```python
from build123d import *

# Parameters (mm, degrees)
SKETCH1_R                = 0.406598389
SKETCH1_R_2              = 1.143
BASE_EXTRUDE_DEPTH       = 6.35
SKETCH2_W                = 2.8702
SKETCH2_H                = 3.81
CUT_EXTRUDE1_DEPTH       = 33.262756347
SKETCH3_W                = 3.302
SKETCH3_H                = 0.508
BOSS_EXTRUDE1_DEPTH      = 3.81
BOSS_EXTRUDE2_DEPTH      = 3.81
SKETCH5_W                = 6.170551723
SKETCH5_H                = 2.54
CUT_EXTRUDE2_DEPTH       = 6.096
SKETCH6_R                = 2.3114
BOSS_EXTRUDE3_DEPTH      = 2.54
BOSS_EXTRUDE4_DEPTH      = 0.254
BOSS_EXTRUDE4_DEPTH_BACK = 4.064
SKETCH7_R                = 0.752584906


with BuildPart() as part:
    # Sketch1 → Base-Extrude (new body)
    with BuildSketch(Plane.XY):
        with BuildLine():
            Line((15.748192067, 1.405399301), (15.748192067, 10.955799301))
            Line((15.748192067, 10.955799301), (15.240192067, 11.463799301))
            Line((15.240192067, 11.463799301), (15.240192067, 14.079999301))
            Line((15.240192067, 14.079999301), (13.131992067, 14.079999301))
            ThreePointArc((13.131992067, 14.079999301), (12.5931767, 14.303183934), (12.369992067, 14.841999301))
            Line((12.369992067, 14.841999301), (12.369992067, 19.718799301))
            ThreePointArc((12.369992067, 19.718799301), (12.5931767, 20.257614668), (13.131992067, 20.480799301))
            Line((13.131992067, 20.480799301), (23.876192067, 20.480799301))
            ThreePointArc((23.876192067, 20.480799301), (24.415007435, 20.257614668), (24.638192067, 19.718799301))
            Line((24.638192067, 19.718799301), (24.638192067, 1.405399301))
            ThreePointArc((24.638192067, 1.405399301), (24.415007435, 0.866583934), (23.876192067, 0.643399301))
            Line((23.876192067, 0.643399301), (16.510192067, 0.643399301))
            ThreePointArc((16.510192067, 0.643399301), (15.9713767, 0.866583934), (15.748192067, 1.405399301))
        make_face()
        with Locations((13.639992067, 18.270999301)):
            Circle(SKETCH1_R, mode=Mode.SUBTRACT)
        with Locations((13.639992067, 15.095999301)):
            Circle(SKETCH1_R, mode=Mode.SUBTRACT)
        with Locations((22.275992067, 5.799599301)):
            Circle(SKETCH1_R_2, mode=Mode.SUBTRACT)
        with BuildLine():
            Line((23.418992067, 15.197599301), (23.418992067, 15.451599301))
            ThreePointArc((23.418992067, 15.451599301), (22.275992067, 16.594599301), (21.132992067, 15.451599301))
            Line((21.132992067, 15.451599301), (21.132992067, 15.197599301))
            ThreePointArc((21.132992067, 15.197599301), (22.275992067, 14.054599301), (23.418992067, 15.197599301))
        make_face(mode=Mode.SUBTRACT)
    extrude(amount=-BASE_EXTRUDE_DEPTH)

    # Sketch2 → Cut-Extrude1 (cut, through all)
    with BuildSketch(Plane(origin=(0, 20.480799301, 0), x_dir=(-1, 0, 0), z_dir=(0, 1, 0))):
        with Locations((-13.805092067, -3.175)):
            Rectangle(SKETCH2_W, SKETCH2_H)
    extrude(amount=-CUT_EXTRUDE1_DEPTH, mode=Mode.SUBTRACT)

    # Sketch3 → Boss-Extrude1 (add)
    with BuildSketch(Plane(origin=(24.638192067, 0, 0), x_dir=(0, 0, -1), z_dir=(1, 0, 0))):
        with Locations((3.175, 18.194799301)):
            Rectangle(SKETCH3_W, SKETCH3_H)
        with Locations((3.175, 8.034799301)):
            Rectangle(SKETCH3_W, SKETCH3_H)
        with Locations((3.175, 2.192799301)):
            Rectangle(SKETCH3_W, SKETCH3_H)
    extrude(amount=BOSS_EXTRUDE1_DEPTH)

    # Sketch4 → Boss-Extrude2 (add)
    with BuildSketch(Plane.XY.offset(-5.08)):
        with BuildLine():
            Line((13.259938371, 19.630855819), (14.196083485, 2.477721783))
            Line((14.196083485, 2.477721783), (11.012636903, 2.291505495))
            ThreePointArc((11.012636903, 2.291505495), (9.341497952, 0.412712637), (11.22029081, -1.258426314))
            Line((11.22029081, -1.258426314), (15.023756731, -1.035345448))
            Line((15.023756731, -1.035345448), (13.893994801, 19.665459923))
            Line((13.893994801, 19.665459923), (13.259938371, 19.630855819))
        make_face()
    extrude(amount=BOSS_EXTRUDE2_DEPTH)

    # Sketch5 → Cut-Extrude2 (cut)
    with BuildSketch(Plane(origin=(-0.096031652, 1.641701906, 0), x_dir=(-0.9982935348358413, -0.05839536201584024, 0), z_dir=(-0.05839536201584024, 0.9982935348358413, 0))):
        with Locations((-11.231269963, -3.175)):
            Rectangle(SKETCH5_W, SKETCH5_H)
    extrude(amount=-CUT_EXTRUDE2_DEPTH, mode=Mode.SUBTRACT)

    # Sketch6 → Boss-Extrude3 (add)
    with BuildSketch(Plane.XY.offset(-4.445)):
        with Locations(Location((11.116463856, 0.51653959, 0), (0, 0, 53.632575023))):
            Circle(SKETCH6_R)
    extrude(amount=BOSS_EXTRUDE3_DEPTH)

    # Sketch7 → Boss-Extrude4 (add, two sides: drawn at the far end of the back side and taken through both)
    with BuildSketch(Plane.XY.offset(-1.27).offset(-BOSS_EXTRUDE4_DEPTH_BACK)):
        with Locations(Location((11.116463856, 0.51653959, 0), (0, 0, 180))):
            Circle(SKETCH7_R)
    extrude(amount=BOSS_EXTRUDE4_DEPTH + BOSS_EXTRUDE4_DEPTH_BACK)


solid = part.part
```
CAD build for the part. Positions are in the model's coordinates, mm. A direction names the side the tool comes from. Round coordinates to 2 decimals unless told otherwise and drop trailing zeros. Order: outer loops, then holes, each group sorted by start corner. A loop starts at its lowest first (then second) coordinate and runs counter-clockwise, first axis right, second up.
Item 1: Mould opens along X. For faces 5 (the face through (13.234, 15.114, -5.706)), 6 (the face through (27, 2.447, -3)), 7 (the face through (12.37, 17, -6)) say: pulls with the +X half, pulls with the -X half, needs draft (parallel to the pull), parting line crosses it, or undercut.
Item 2: Pin check, flat tips, straight feed: pin 1 (1.8 mm diameter, centred on x = 22.28, y = 5.8, fed in from -Z); pin 2 (3.5 mm diameter, centred on x = 27.5, z = -3.5, fed in from +Y); pin 3 (0.6 mm diameter, centred on y = 17, z = -0.5, fed in from -X); pin 4 (1.7 mm diameter, centred on x = 26.5, z = -2.5, fed in from -Y). Stop position of each tip, or through.
Item 3: Probe line 1 along X through (y, z) = (14.75, -2.75); line 2 along X through (y, z) = (14.5, -4.5); line 3 along Y through (x, z) = (22.25, -1). List the from-to ranges inside material, lowest first.
Item 4: Saw through at A-A on x = 27.25. Write the cut outline in (y, z), then the cut area to 3 significant figures.
Item 5: Saw through at C-C on y = 6.5. Write the cut outline in (x, z), then the cut area to 3 significant figures.
Item 6: Saw through at D-D on y = 17.5. Write the cut outline in (x, z).
Item 7: Saw through at B-B on z = -4. State how many separate pieces and enclosed holes the cut face has, then the cut area to 3 significant figures.
Item 8: Tool access for faces 1 (the face through (14, 14.08, -6)), 2 (the face through (27, 18.449, -3)), 3 (the face through (14.3, 0.7, -3.2)), 4 (the face through (27, 7.781, -3)): list every direction of +Z, -Z, +X, -X, +Y, -Y with a clear straight run to the whole face (end or side of a thin tool).
Reported:
1. face 5: undercut
1. face 6: needs draft
1. face 7: pulls with the -X half
2. pin 1: passes through
2. pin 2: stops at y = 18.45
2. pin 3: stops at x = 12.37
2. pin 4: stops at y = 1.94
3. line 1: x = 13.53 to 14.16, 15.24 to 21.22, 23.33 to 24.64
3. line 2: x = 13.54 to 14.18, 15.24 to 21.37, 23.18 to 24.64
3. line 3: y = 0.64 to 4.66, 6.94 to 14.05, 16.59 to 20.48
4. outline: (1.94, -4.83) - (2.45, -4.83) - (2.45, -1.52) - (1.94, -1.52) - close; (7.78, -4.83) - (8.29, -4.83) - (8.29, -1.52) - (7.78, -1.52) - close; (17.94, -4.83) - (18.45, -4.83) - (18.45, -1.52) - (17.94, -1.52) - close
4. area: 5.03 mm2
5. outline: (13.98, -5.08) - (14.61, -5.08) - (14.61, -1.27) - (13.98, -1.27) - close; (15.75, -6.35) - (21.37, -6.35) - (21.37, 0) - (15.75, 0) - close; (23.18, -6.35) - (24.64, -6.35) - (24.64, 0) - (23.18, 0) - close
5. area: 47.4 mm2
6. outline: (12.37, -6.35) - (24.64, -6.35) - (24.64, 0) - (12.37, 0) - (12.37, -1.27) - (13.38, -1.27) - (13.38, -5.08) - (12.37, -5.08) - close; hole (14.01, -5.08) - (15.24, -5.08) - (15.24, -1.27) - (14.01, -1.27) - close
7. separate pieces: 3
7. enclosed holes: 2
7. area: 208 mm2
8. face 1: -Z, -X, -Y
8. face 2: +Z, -Z, +X, +Y
8. face 3: -Y
8. face 4: +Z, -Z, +X
